Study the drawing (mm; zero at the part's minimum x, y, z) and answer. Coordinates: 2 decimals unless noted, no trailing zeros. Loops run counter-clockwise (first coordinate to the right, second up) from the corner with the lowest first, then second, coordinate; pieces in that order, holes last.
Q1. Straight lines are drawn through the part: line 1 (Z direction, x = 30, y = 0.15); line 2 (X direction, y = 0.65, z = 12.25); line 3 (X direction, y = 0.9, z = 5). For each, find the intervals that lie inside material, in ascending order.
Q2. Section C-C (y = 0.85) is taken. Give the vertices of the cut face in (x, z), then the cut area to 3 significant figures.
Q3. Section B-B (z = 5.25) is taken. Give the vertices of the cut face in (x, y), then the cut area to 3 significant figures.
Q4. Section D-D (z = 12.25) is taken. Give the vertices of the cut face in (x, y).
Q5. The mould has two halves that part along Y. Classify the marked faces 1 and 2: pulls with the +Y half, pulls with the -Y half, needs draft (parallel to the pull), parting line crosses it, or undercut.
Q6. Section A-A (x = 42.5) is taken. Give the vertices of the cut face in (y, z), then the cut area to 3 significant figures.
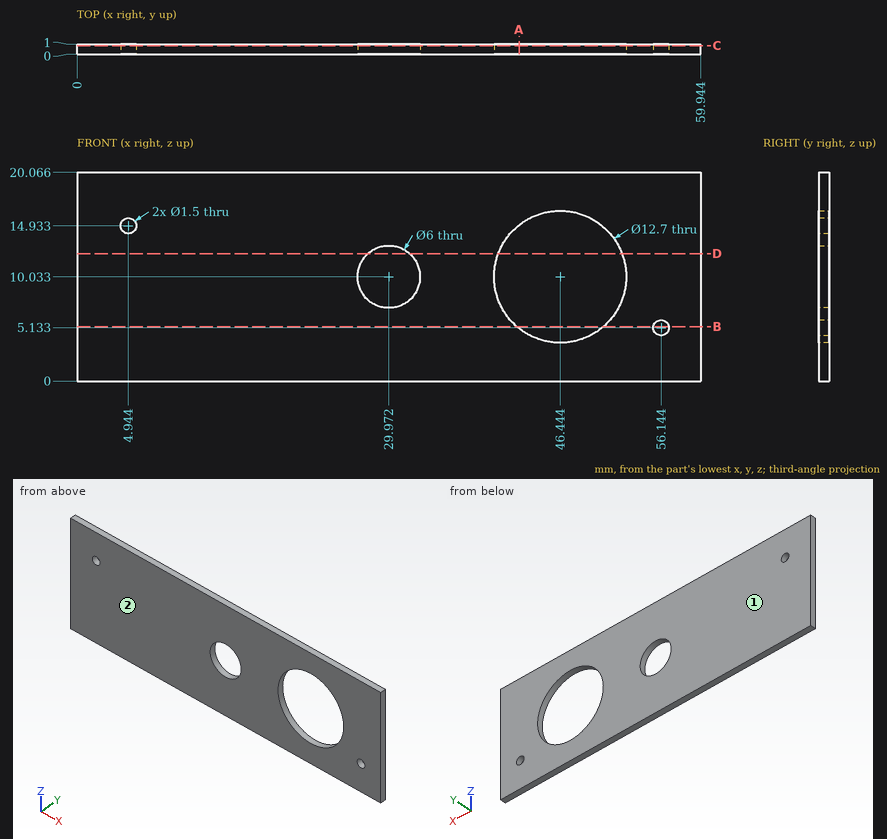
Numbers:
1. line 1: z = 0 to 7.03, 13.03 to 20.07
1. line 2: x = 0 to 27.95, 31.99 to 40.49, 52.39 to 59.94
1. line 3: x = 0 to 42.57, 50.32 to 55.41, 56.88 to 59.94
2. outline: (0, 0) - (59.94, 0) - (59.94, 20.07) - (0, 20.07) - close; hole circle Ø1.5 at (4.94, 14.93); hole circle Ø6 at (29.97, 10.03); hole circle Ø12.7 at (46.44, 10.03); hole circle Ø1.5 at (56.14, 5.13)
2. area: 1,040 mm2
3. outline: (0, 0) - (42.27, 0) - (42.27, 1) - (0, 1) - close; (50.62, 0) - (55.4, 0) - (55.4, 1) - (50.62, 1) - close; (56.88, 0) - (59.94, 0) - (59.94, 1) - (56.88, 1) - close
3. area: 50.1 mm2
4. outline: (0, 0) - (27.95, 0) - (27.95, 1) - (0, 1) - close; (31.99, 0) - (40.49, 0) - (40.49, 1) - (31.99, 1) - close; (52.39, 0) - (59.94, 0) - (59.94, 1) - (52.39, 1) - close
5. face 1: pulls with the +Y half
5. face 2: pulls with the -Y half
6. outline: (0, 0) - (1, 0) - (1, 5.06) - (0, 5.06) - close; (0, 15.01) - (1, 15.01) - (1, 20.07) - (0, 20.07) - close
6. area: 10.1 mm2
